```python
from build123d import *

# Parameters (mm, degrees)
F0_R     = 7.95
F1_DEPTH = 3
F2_R     = 8.75
F3_DEPTH = 3.5
F4_R     = 7.95
F5_DEPTH = 3
F7_DEPTH = 25
F6_R     = 1.2
F8_DEPTH = 7


with BuildPart() as f1:
    # F0 (on Top) → F1 (new body)
    with BuildSketch(Plane.XY):
        Circle(F0_R)
    extrude(amount=F1_DEPTH)

    # F2 (on face) → F3 (join)
    with BuildSketch(Plane.XY.offset(3)):
        Circle(F2_R)
    extrude(amount=F3_DEPTH)

    # F4 (on face) → F5 (join)
    with BuildSketch(Plane.XY.offset(6.5)):
        Circle(F4_R)
    extrude(amount=F5_DEPTH)

    # F6 (on face) → F7 (cut)
    with BuildSketch(Plane.XY.offset(9.5)):
        with BuildLine():
            ThreePointArc((-2.598076, 1.5), (-2.458255, 1.719588), (-2.299923, 1.926228))
            Line((-2.299923, 1.926228), (-2.915072, 6.243758))
            ThreePointArc((-2.915072, 6.243758), (-4.883769, 4.86117), (-6.257211, 2.886082))
            Line((-6.257211, 2.886082), (-2.598076, 1.5))
        make_face()
        with BuildLine():
            ThreePointArc((0, 3), (0.26008, 2.988705), (0.518201, 2.954906))
            Line((0.518201, 2.954906), (3.949717, 5.646406))
            ThreePointArc((3.949717, 5.646406), (1.768012, 6.660052), (-0.629185, 6.861945))
            Line((-0.629185, 6.861945), (0, 3))
        make_face()
        with BuildLine():
            ThreePointArc((2.598076, 1.5), (2.718334, 1.269117), (2.818124, 1.028678))
            Line((2.818124, 1.028678), (6.864789, -0.597352))
            ThreePointArc((6.864789, -0.597352), (6.884242, -0.298958), (6.89073, 0))
            ThreePointArc((6.89073, 0), (6.567472, 2.08578), (5.628026, 3.975863))
            Line((5.628026, 3.975863), (2.598076, 1.5))
        make_face()
        with BuildLine():
            Line((6.257211, -2.886082), (2.598076, -1.5))
            ThreePointArc((2.598076, -1.5), (2.458255, -1.719588), (2.299923, -1.926228))
            Line((2.299923, -1.926228), (2.915072, -6.243758))
            ThreePointArc((2.915072, -6.243758), (4.883769, -4.86117), (6.257211, -2.886082))
        make_face()
        with BuildLine():
            Line((0.629185, -6.861945), (0, -3))
            ThreePointArc((0, -3), (-0.26008, -2.988705), (-0.518201, -2.954906))
            Line((-0.518201, -2.954906), (-3.949717, -5.646406))
            ThreePointArc((-3.949717, -5.646406), (-1.768012, -6.660052), (0.629185, -6.861945))
        make_face()
        with BuildLine():
            Line((-5.628026, -3.975863), (-2.598076, -1.5))
            ThreePointArc((-2.598076, -1.5), (-2.718334, -1.269117), (-2.818124, -1.028678))
            Line((-2.818124, -1.028678), (-6.864789, 0.597352))
            ThreePointArc((-6.864789, 0.597352), (-6.651781, -1.798883), (-5.628026, -3.975863))
        make_face()
    extrude(amount=-F7_DEPTH, mode=Mode.SUBTRACT)

    # F6 (on face) → F8 (cut)
    with BuildSketch(Plane.XY.offset(9.5)):
        Circle(F6_R)
        with BuildLine():
            ThreePointArc((-2.818124, -1.028678), (-2.988705, 0.26008), (-2.598076, 1.5))
            Line((-2.598076, 1.5), (-6.257211, 2.886082))
            ThreePointArc((-6.257211, 2.886082), (-6.660052, 1.768012), (-6.864789, 0.597352))
            Line((-6.864789, 0.597352), (-2.818124, -1.028678))
        make_face()
        with BuildLine():
            ThreePointArc((-2.299923, 1.926228), (-1.269117, 2.718334), (0, 3))
            Line((0, 3), (-0.629185, 6.861945))
            ThreePointArc((-0.629185, 6.861945), (-1.798883, 6.651781), (-2.915072, 6.243758))
            Line((-2.915072, 6.243758), (-2.299923, 1.926228))
        make_face()
        with BuildLine():
            ThreePointArc((0.518201, 2.954906), (1.719588, 2.458255), (2.598076, 1.5))
            Line((2.598076, 1.5), (5.628026, 3.975863))
            ThreePointArc((5.628026, 3.975863), (4.86117, 4.883769), (3.949717, 5.646406))
            Line((3.949717, 5.646406), (0.518201, 2.954906))
        make_face()
        with BuildLine():
            ThreePointArc((2.818124, 1.028678), (2.954181, 0.522316), (3, 0))
            ThreePointArc((3, 0), (2.897777, -0.776457), (2.598076, -1.5))
            Line((2.598076, -1.5), (6.257211, -2.886082))
            ThreePointArc((6.257211, -2.886082), (6.660052, -1.768012), (6.864789, -0.597352))
            Line((6.864789, -0.597352), (2.818124, 1.028678))
        make_face()
        with BuildLine():
            Line((2.915072, -6.243758), (2.299923, -1.926228))
            ThreePointArc((2.299923, -1.926228), (1.269117, -2.718334), (0, -3))
            Line((0, -3), (0.629185, -6.861945))
            ThreePointArc((0.629185, -6.861945), (1.798883, -6.651781), (2.915072, -6.243758))
        make_face()
        with BuildLine():
            Line((-3.949717, -5.646406), (-0.518201, -2.954906))
            ThreePointArc((-0.518201, -2.954906), (-1.719588, -2.458255), (-2.598076, -1.5))
            Line((-2.598076, -1.5), (-5.628026, -3.975863))
            ThreePointArc((-5.628026, -3.975863), (-4.86117, -4.883769), (-3.949717, -5.646406))
        make_face()
    extrude(amount=-F8_DEPTH, mode=Mode.SUBTRACT)


solid = f1.part
```
Could you check a few things on this model? Use its own coordinates, in mm. A direction names the side the tool comes from. Coordinates: 2 decimals unless noted, no trailing zeros. Order: outer loops, then holes, each group sorted by start corner. A loop starts at its lowest first (then second) coordinate and runs counter-clockwise, first axis right, second up. Notation, with made-up numbers: M 51,78 L 107,78 A18 cw 107,110 Z; hole C 67.25,65.5 d2. An arc over 180 degrees is marked long. Use a Markdown table: item, result. Add a question column.
Q1. I want a section at A-A on z = 2.75. List the corners of the cut face in (x, y) for me.
Q2. I want a section at D-D on y = -5. List the corners of the cut face in (x, z) for me, then the cut area to 3 significant figures.
Q3. I'm going to push flat-ended pins straight in: pin 1 (4 mm diameter, centred on x = -5, z = 2.5, fed in from +Y); pin 2 (1 mm diameter, centred on x = -3, y = -4, fed in from +Z); pin 3 (3 mm diameter, centred on y = -5, z = 6.5, fed in from -X). Where does each tip first touch, or does it pass through?
Q4. I want a section at C-C on z = 1. List the corners of the cut face in (x, y) for me, then the cut area to 3 significant figures.
Q5. If I drill on L1, parallel to X at y = 1, z = 8; L2, parallel to X at y = -0.5, z = 5.5; L3, parallel to Z at x = -6.25, y = 2, over which ranges is the centre line in solid material (lowest first)?
Q6. Which directions (+Z, -Z, +X, -X, +Y, -Y) give clear straight access to the entire face, cutting with the end or side of a thin tool? Please do faces 1 (the cylindrical face through (-1.72, -7.76, 7.98)), 2 (the flat face through (-4.45, 2.2, 1.27)).
Q7. I want a section at B-B on x = 2. List the corners of the cut face in (y, z) for me, then the cut area to 3 significant figures.
Q8. We'd pull the mould along X, two halves only. Please class faces 3 (the cylindrical face through (-1.72, -7.76, 1.48)), 4 (the flat face through (-2.21, -4.28, 1.27)), 5 (the flat face through (-0.32, 4.96, 1.27)), 6 (the flat face through (0, 0, 0)): pulls with the +X half, pulls with the -X half, needs draft (parallel to the pull), parting line crosses it, or undercut.
Checked values:
| question | item | result |
|---|---|---|
| 1 | outline | C 0,0 d15.9; M -2.82,-1.03 A3 ccw -2.6,-1.5 A3 ccw -0.52,-2.95 A3 ccw 0,-3 A3 ccw 2.3,-1.93 A3 ccw 2.6,-1.5 A3 ccw 3,0 A3 ccw 2.82,1.03 A3 ccw 2.6,1.5 A3 ccw 0.52,2.95 A3 ccw 0,3 A3 ccw -2.3,1.93 A3 ccw -2.6,1.5 A3 ccw Z; hole M -6.86,0.6 A6.89 ccw -5.63,-3.98 A6.89 ccw -3.95,-5.65 A6.89 ccw 0.63,-6.86 A6.89 ccw 2.92,-6.24 A6.89 ccw 6.26,-2.89 A6.89 ccw 6.86,-0.6 A6.89 ccw 6.89,0 A6.89 ccw 5.63,3.98 A6.89 ccw 3.95,5.65 A6.89 ccw -0.63,6.86 A6.89 ccw -2.92,6.24 A6.89 ccw -6.26,2.89 A6.89 ccw Z; hole C 0,0 d2.4 |
| 2 | outline | M -7.18,3 L -6.18,3 L -6.18,0 L -3.13,0 L -3.13,2.5 L -4.74,2.5 L -4.74,9.5 L -6.18,9.5 L -6.18,6.5 L -7.18,6.5 Z; M 0.33,0 L 2.74,0 L 2.74,2.5 L 0.33,2.5 Z; M 4.74,0 L 6.18,0 L 6.18,3 L 7.18,3 L 7.18,6.5 L 6.18,6.5 L 6.18,9.5 L 4.74,9.5 Z |
| 2 | area | 44.4 mm² |
| 3 | pin 1 | y = 8.2 |
| 3 | pin 2 | z = 2.5 |
| 3 | pin 3 | x = -8.02 |
| 4 | outline | C 0,0 d15.9; hole M -6.86,0.6 A6.89 ccw -5.63,-3.98 L -2.6,-1.5 A3 cw -2.82,-1.03 Z; hole M -6.26,2.89 L -2.6,1.5 A3 cw -2.3,1.93 L -2.92,6.24 A6.89 ccw Z; hole M -3.95,-5.65 A6.89 ccw 0.63,-6.86 L 0,-3 A3 cw -0.52,-2.95 Z; hole M -0.63,6.86 L 0,3 A3 cw 0.52,2.95 L 3.95,5.65 A6.89 ccw Z; hole M 2.3,-1.93 L 2.92,-6.24 A6.89 ccw 6.26,-2.89 L 2.6,-1.5 A3 cw Z; hole M 2.6,1.5 A3 cw 2.82,1.03 L 6.86,-0.6 A6.89 ccw 6.89,0 A6.89 ccw 5.63,3.98 Z |
| 4 | area | 135 mm² |
| 5 | L1 | -7.89 to -6.82, -2.83 to -0.66, 0.66 to 2.83, 6.82 to 7.89 |
| 5 | L2 | -8.74 to -6.87, -2.96 to -1.09, 1.09 to 2.96, 6.87 to 8.74 |
| 5 | L3 | 0 to 2.5 |
| 6 | face 1 | +Z |
| 6 | face 2 | +Z, -Z |
| 7 | outline | M -8.52,3 L -7.69,3 L -7.69,0 L 4.12,0 L 4.12,2.5 L 2.24,2.5 L 2.24,9.5 L -2.24,9.5 L -2.24,2.5 L -6.59,2.5 L -6.59,9.5 L -7.69,9.5 L -7.69,6.5 L -8.52,6.5 Z; M 6.59,0 L 7.69,0 L 7.69,3 L 8.52,3 L 8.52,6.5 L 7.69,6.5 L 7.69,9.5 L 6.59,9.5 Z |
| 7 | area | 84.8 mm² |
| 8 | face 3 | parting line crosses it |
| 8 | face 4 | undercut |
| 8 | face 5 | undercut |
| 8 | face 6 | needs draft |
